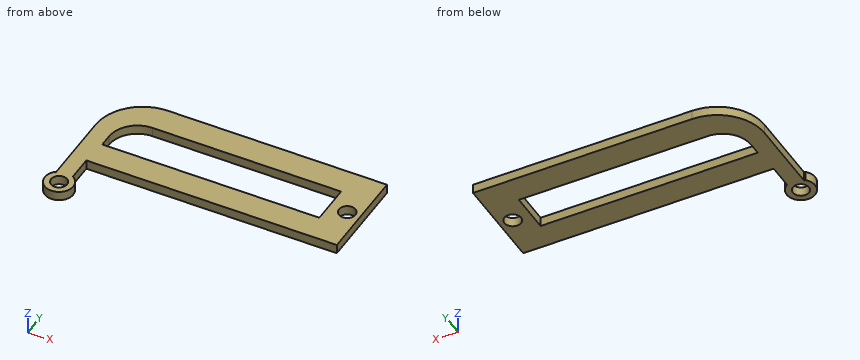
from build123d import *

# Parameters (mm, degrees)
SKETCH1_R           = 1.7
SKETCH1_R_2         = 1.75
BOSS_EXTRUDE2_DEPTH = 2
FILLET1_R           = 10
CUT_EXTRUDE1_DEPTH  = 4.3


with BuildPart() as part:
    # Sketch1 → Boss-Extrude2 (new body)
    with BuildSketch(Plane.XY):
        with BuildLine():
            Line((-24.301399152, -6.742575532), (21.488241451, -6.742575532))
            Line((21.488241451, -6.742575532), (28.630568437, -6.742575532))
            Line((28.630568437, -6.742575532), (28.630568437, 13.257424468))
            Line((28.630568437, 13.257424468), (21.488241451, 13.257424468))
            Line((21.488241451, 13.257424468), (-17.840083641, 13.257424468))
            Line((-17.840083641, 13.257424468), (-21.005321996, 13.257424468))
            Line((-21.005321996, 13.257424468), (-27.697276817, 13.257424468))
            Line((-27.697276817, 13.257424468), (-27.697276817, -12.486730567))
            Line((-27.697276817, -12.486730567), (-27.960658237, -12.486730567))
            ThreePointArc((-27.960658237, -12.486730567), (-25.553021513, -17.62663418), (-24.301399152, -12.090501486))
            Line((-24.301399152, -12.090501486), (-24.301399152, -8.994116068))
            Line((-24.301399152, -8.994116068), (-24.301399152, -6.742575532))
        make_face()
        with Locations((-25.875977425, -14.644068258)):
            Circle(SKETCH1_R, mode=Mode.SUBTRACT)
        with Locations((25.830760295, 2.700271972)):
            Circle(SKETCH1_R_2, mode=Mode.SUBTRACT)
    extrude(amount=BOSS_EXTRUDE2_DEPTH)

    # Fillet1
    fillet1_edges = [part.edges().sort_by_distance(p)[0] for p in [
        (-27.697276817, 13.257424468, 1),
    ]]
    fillet(fillet1_edges, radius=FILLET1_R)

    # Sketch2 → Cut-Extrude1 (cut)
    with BuildSketch(Plane.XY.offset(2)):
        with BuildLine():
            Line((-23.863033574, -1.206587224), (22.005338697, -1.206587224))
            Line((22.005338697, -1.206587224), (22.005338697, 7.467544216))
            Line((22.005338697, 7.467544216), (-17.863033574, 7.467544216))
            ThreePointArc((-17.863033574, 7.467544216), (-22.105674261, 5.710184903), (-23.863033574, 1.467544216))
            Line((-23.863033574, 1.467544216), (-23.863033574, -1.206587224))
        make_face()
    extrude(amount=-CUT_EXTRUDE1_DEPTH, mode=Mode.SUBTRACT)


solid = part.part
Input: part model. Units: mm. Frame: model coordinates. Give positions to 0.01 mm unless a question says otherwise; leave off trailing zeros. Write each loop counter-clockwise with the first axis right and the second up, starting at its lowest first coordinate (ties: lowest second). Pieces come first, ordered by that corner, then holes. Notation, with made-up numbers: M 28,68 L 53,68 A27 cw 53,92 Z; hole C 6.25,48 d9. An arc over 180 degrees is marked long. Write item = value, one per line. Start each with the question number.
1) Cut plane A-A on x = 18.5. Return the cut outline in (y, z).
2) Material intervals for line 1 along Y through (x, z) = (-15, 1.5); line 2 along X through (y, z) = (-6, 0.15); line 3 along Y through (x, z) = (-24.5, 1.1), sorted ascending. Write a range as [from, to].
3) Cut plane C-C on y = 6. Return the cut outline in (x, z), then the cut area to 3 significant figures.
4) First-contact query: pin 1 Ø4.5 at (x, y) = (-25.88, -14.64) entering from -Z; pin 2 Ø0.6 at (x, z) = (8, 0.5) entering from -Y; pin 3 Ø1 at (y, z) = (-7, 1) entering from -X. Flat tips, straight axial feed; report the tip coordinate or a pass-through.
5) Cut plane D-D on y = -3.5. Return the cut outline in (x, z), then the cut area to 3 significant figures.
6) Cut plane B-B on z = 0.65. Return the cut outline in (x, y).
Solved:
q1.outline = M -6.74,0 L -1.21,0 L -1.21,2 L -6.74,2 Z; M 7.47,0 L 13.26,0 L 13.26,2 L 7.47,2 Z
q2.line_1 = [-6.74, -1.21], [7.47, 13.26]
q2.line_2 = [-27.7, 28.63]
q2.line_3 = [-17.31, -15.64], [-13.65, 10.59]
q3.outline = M -27.31,0 L -21.79,0 L -21.79,2 L -27.31,2 Z; M 22.01,0 L 28.63,0 L 28.63,2 L 22.01,2 Z
q3.area = 24.3 mm2
q4.pin_1 = 0
q4.pin_2 = -6.74
q4.pin_3 = -27.7
q5.outline = M -27.7,0 L 28.63,0 L 28.63,2 L -27.7,2 Z
q5.area = 113 mm2
q6.outline = M -27.96,-12.49 A3 ccw long -24.3,-12.09 L -24.3,-6.74 L 28.63,-6.74 L 28.63,13.26 L -17.7,13.26 A10 ccw -27.7,3.26 L -27.7,-12.49 Z; hole C -25.88,-14.64 d3.4; hole M -23.86,-1.21 L 22.01,-1.21 L 22.01,7.47 L -17.86,7.47 A6 ccw -23.86,1.47 Z; hole C 25.83,2.7 d3.5
